```python
from build123d import *

# Parameters (mm, degrees)
SKETCH1_R                = 37.5
BOSS_EXTRUDE1_DEPTH      = 7.6
CUT_EXTRUDE2_START       = -7.6
CUT_EXTRUDE2_DEPTH       = 7.6
SKETCH4_R                = 45
SKETCH4_R_2              = 37.5
BOSS_EXTRUDE2_DEPTH      = 7.6
SKETCH6_R                = 45
BOSS_EXTRUDE3_DEPTH      = 2
SKETCH7_R                = 1.75
CUT_EXTRUDE3_DEPTH       = 65.359614666
CIRPATTERN2_COUNT        = 3
CUT_EXTRUDE7_DEPTH       = 65.359614666
FILLET3_R                = 1
CIRPATTERN3_COUNT        = 3
FILLET3_OF_CIRPATTERN3_R = 1
BOSS_EXTRUDE4_START      = 1.8
SKETCH15_R               = 1.75
BOSS_EXTRUDE4_DEPTH      = 1.8
CIRPATTERN4_COUNT        = 3


# Read off the part's stored shape, not the designer's step: Cut-Extrude2
with BuildPart() as part:
    # Sketch1 → Boss-Extrude1 (new body)
    with BuildSketch(Plane(origin=(0, 0, 0), x_dir=(1, 0, 0), z_dir=(0, 1, 0))):
        with Locations(Location((0, 0, 0), (0, 0, 90))):
            Circle(SKETCH1_R)
    extrude(amount=BOSS_EXTRUDE1_DEPTH)

    # Cut-Extrude2 outline → Cut-Extrude2 (cut)
    with BuildSketch(Plane(origin=(0, 7.6, 0), x_dir=(1, 0, 0), z_dir=(0, 1, 0)).offset(CUT_EXTRUDE2_START)):
        with BuildLine():
            ThreePointArc((-24.104535363, -28.726666617), (0, -24.760936498), (24.104535363, -28.726666617))
            ThreePointArc((24.104535363, -28.726666617), (32.475952642, -18.75), (36.930290738, -6.511806663))
            ThreePointArc((36.930290738, -6.511806663), (21.443600029, 12.380468249), (12.825755375, 35.238473279))
            ThreePointArc((12.825755375, 35.238473279), (0, 37.5), (-12.825755375, 35.238473279))
            ThreePointArc((-12.825755375, 35.238473279), (-21.443600029, 12.380468249), (-36.930290738, -6.511806663))
            ThreePointArc((-36.930290738, -6.511806663), (-32.475952642, -18.75), (-24.104535363, -28.726666617))
        make_face()
    extrude(amount=CUT_EXTRUDE2_DEPTH, mode=Mode.SUBTRACT)

    # Sketch4 → Boss-Extrude2 (add)
    with BuildSketch(Plane(origin=(0, 0, 0), x_dir=(1, 0, 0), z_dir=(0, 1, 0))):
        with Locations(Location((0, 0, 0), (0, 0, 90))):
            Circle(SKETCH4_R)
        Circle(SKETCH4_R_2, mode=Mode.SUBTRACT)
    extrude(amount=BOSS_EXTRUDE2_DEPTH)

    # Sketch6 → Boss-Extrude3 (add)
    with BuildSketch(Plane(origin=(0, 7.6, 0), x_dir=(1, 0, 0), z_dir=(0, 1, 0))):
        with Locations(Location((0, 0, 0), (0, 0, 90))):
            Circle(SKETCH6_R)
        with BuildLine():
            ThreePointArc((-28.952849653, 1.653026611), (-25.11473671, -14.5), (-13.044861788, -25.900416617))
            ThreePointArc((-13.044861788, -25.900416617), (0, -24.760936498), (13.044861788, -25.900416617))
            ThreePointArc((13.044861788, -25.900416617), (25.11473671, -14.5), (28.952849653, 1.653026611))
            ThreePointArc((28.952849653, 1.653026611), (21.443600029, 12.380468249), (15.907987865, 24.247390006))
            ThreePointArc((15.907987865, 24.247390006), (0, 29), (-15.907987865, 24.247390006))
            ThreePointArc((-15.907987865, 24.247390006), (-21.443600029, 12.380468249), (-28.952849653, 1.653026611))
        make_face(mode=Mode.SUBTRACT)
    extrude(amount=BOSS_EXTRUDE3_DEPTH)

    # Sketch7 → Cut-Extrude3 (cut, through all)
    with BuildSketch(Plane(origin=(0, 9.6, 0), x_dir=(1, 0, 0), z_dir=(0, 1, 0))):
        with Locations(Location((0, 32, 0), (0, 0, 270))):
            Circle(SKETCH7_R)
    cut_extrude3 = extrude(amount=-CUT_EXTRUDE3_DEPTH, mode=Mode.SUBTRACT)

    # CirPattern2: Cut-Extrude3 ×3 about axis
    cirpattern2_axis = Axis((0, 0, 0), (0, 1, 0))
    for i in range(1, CIRPATTERN2_COUNT):
        add(cut_extrude3.rotate(cirpattern2_axis, i * 360 / CIRPATTERN2_COUNT), mode=Mode.SUBTRACT)

    # Sketch13 → Cut-Extrude7 (cut, through all)
    with BuildSketch(Plane.XZ):
        with BuildLine():
            ThreePointArc((-22.11228446, 33.332369792), (0, 29.760936498), (22.11228446, 33.332369792))
            ThreePointArc((22.11228446, 33.332369792), (0, 40), (-22.11228446, 33.332369792))
        make_face()
    cut_extrude7 = extrude(amount=-CUT_EXTRUDE7_DEPTH, mode=Mode.SUBTRACT)

    # Fillet3
    fillet3_edges = [part.edges().sort_by_distance(p)[0] for p in [
        (-22.11228446, 4.8, 33.332369792),
        (22.11228446, 4.8, 33.332369792),
    ]]
    fillet(fillet3_edges, radius=FILLET3_R)

    # CirPattern3: Cut-Extrude7 ×3 about axis
    cirpattern3_axis = Axis((0, 0, 0), (0, 1, 0))
    for i in range(1, CIRPATTERN3_COUNT):
        add(cut_extrude7.rotate(cirpattern3_axis, i * 360 / CIRPATTERN3_COUNT), mode=Mode.SUBTRACT)

    # Fillet3 of CirPattern3
    fillet3_of_cirpattern3_edges = [part.edges().sort_by_distance(p)[0] for p in [
        (39.922821238, 4.8, 2.483615182),
        (17.810536778, 4.8, -35.815984974),
        (-17.810536778, 4.8, -35.815984974),
        (-39.922821238, 4.8, 2.483615182),
    ]]
    fillet(fillet3_of_cirpattern3_edges, radius=FILLET3_OF_CIRPATTERN3_R)

    # Sketch15 → Boss-Extrude4 (add)
    with BuildSketch(Plane.XZ.offset(-7.6).offset(BOSS_EXTRUDE4_START)):
        with BuildLine():
            ThreePointArc((-15.374943027, -25.760650747), (0, -30), (15.374943027, -25.760650747))
            ThreePointArc((15.374943027, -25.760650747), (13.94564115, -30.457951205), (12.825755375, -35.238473279))
            ThreePointArc((12.825755375, -35.238473279), (0, -37.5), (-12.825755375, -35.238473279))
            ThreePointArc((-12.825755375, -35.238473279), (-13.94564115, -30.457951205), (-15.374943027, -25.760650747))
        make_face()
        with Locations(Location((0, -32, 0), (0, 0, 90))):
            Circle(SKETCH15_R, mode=Mode.SUBTRACT)
    boss_extrude4 = extrude(amount=-BOSS_EXTRUDE4_DEPTH)

    # CirPattern4: Boss-Extrude4 ×3 about axis
    cirpattern4_axis = Axis((0, 7.6, 0), (0, -1, 0))
    for i in range(1, CIRPATTERN4_COUNT):
        add(boss_extrude4.rotate(cirpattern4_axis, i * 360 / CIRPATTERN4_COUNT))


solid = part.part
```
Verification items for the finished model (mm, model axes). A direction names the side the tool comes from. Give positions to 0.01 mm unless a question says otherwise; leave off trailing zeros. Order: outer loops, then holes, each group sorted by start corner. A loop starts at its lowest first (then second) coordinate and runs counter-clockwise, first axis right, second up. Notation, with made-up numbers: (72.25, -11.5) -> (121.25, -11.5) arc R18 cw to (121.25, 23.5) -> close; hole circle Ø10 at (41, -6). An arc over 180 degrees is marked (long way). One line per item, written item: value.
(1) Sectioned sample at C-C on x = -32. Record the cut outline in (y, z).
Final values:
outline: (0, -31.64) -> (9.6, -31.64) -> (9.6, -24) -> (0, -24) -> close; (0, -5.82) -> (9.6, -5.82) -> (9.6, 31.64) -> (0, 31.64) -> (0, 19.55) -> (5.8, 19.55) -> (5.8, 1.76) -> (0, 1.76) -> close
(2) Sectioned sample at D-D on z = 20.5. Record the cut outline in (x, y).
Final values:
outline: (-40.06, 0) -> (-31.4, 0) -> (-31.4, 5.8) -> (-21.9, 5.8) -> (-21.9, 7.6) -> (-20.51, 7.6) -> (-20.51, 9.6) -> (-40.06, 9.6) -> close; (20.51, 7.6) -> (21.9, 7.6) -> (21.9, 5.8) -> (31.4, 5.8) -> (31.4, 0) -> (40.06, 0) -> (40.06, 9.6) -> (20.51, 9.6) -> close
(3) Gauge pin test, flat ends, axial feed: pin 1 (6 mm diameter, centred on x = 4.5, z = -29, fed in from -Y); pin 2 (1 mm diameter, centred on x = -23, y = 8.5, fed in from -Z); pin 3 (4 mm diameter, centred on x = -35, y = 7, fed in from +Z). Record the tip position at first contact, or that the pin passes through.
Final values:
pin 1: y = 5.8
pin 2: z = -38.97
pin 3: z = 30.59
(4) Tool access check on faces 1 (the face through (0, 0, 27)), 2 (the face through (0, 5, 40)), 3 (the face through (-25.867, 6.687, 15.195)). Record the directions out of +Z, -Z, +X, -X, +Y, -Y that give a thin tool (end or side, any length) a straight path to the whole face; none if there is none.
Final values:
face 1: +Z, -Z, +X, -X, -Y
face 2: +Y, -Y
face 3: -Y
(5) Sectioned sample at A-A on x = 0. Record the cut outline in (y, z).
Final values:
outline: (0, -45) -> (9.6, -45) -> (9.6, -33.75) -> (5.8, -33.75) -> (5.8, -37.5) -> (0, -37.5) -> close; (0, 24.76) -> (9.6, 24.76) -> (9.6, 29.76) -> (0, 29.76) -> close; (0, 40) -> (9.6, 40) -> (9.6, 45) -> (0, 45) -> close; (5.8, -30.25) -> (9.6, -30.25) -> (9.6, -29) -> (7.6, -29) -> (7.6, -30) -> (5.8, -30) -> close
(6) Sectioned sample at B-B on z = -32. Record the cut outline in (x, y).
Final values:
outline: (-31.64, 0) -> (-24, 0) -> (-24, 9.6) -> (-31.64, 9.6) -> close; (-18.71, 0) -> (-13.55, 0) -> (-13.55, 5.8) -> (-1.75, 5.8) -> (-1.75, 9.6) -> (-18.71, 9.6) -> close; (1.75, 5.8) -> (13.55, 5.8) -> (13.55, 0) -> (18.71, 0) -> (18.71, 9.6) -> (1.75, 9.6) -> close; (24, 0) -> (31.64, 0) -> (31.64, 9.6) -> (24, 9.6) -> close
(7) Scan lines: line 1 along X through (y, z) = (8.75, -23); line 2 along X through (y, z) = (2, -1.5) (3 decimals); line 3 along Z through (x, y) = (-10, 3). Record each from-to range of solid material in increasing order. Write a range as [from, to].
Final values:
line 1: [-38.68, -32.73], [-21.76, -16.37], [16.37, 21.76], [32.73, 38.68]
line 2: [-44.975, -39.972], [-35.796, -29.082], [29.082, 35.796], [39.972, 44.975]
line 3: [-43.87, -36.14], [25.43, 30.48], [38.73, 43.87]
(8) Draft check along Z on faces 4 (the face through (19, 9.6, -19)), 5 (the face through (-32.57, 2.86, 18.59)). Enter one of: pulls with the +Z half, pulls with the -Z half, needs draft (parallel to the pull), parting line crosses it, or undercut.
Final values:
face 4: needs draft
face 5: undercut
